The listing builds one solid part. Answer for the finished solid, in the listing's coordinates (mm). Face numbers are marked on the shaded views. A direction names the side the tool comes from. Coordinates: 2 decimals unless noted, no trailing zeros. Loops run counter-clockwise (first coordinate to the right, second up) from the corner with the lowest first, then second, coordinate; pieces in that order, holes last. Notation, with made-up numbers: (52, 12) - (94, 12) arc R23 ccw to (94, 34) - close; hole circle Ø5 at (28, -35). An arc over 180 degrees is marked (long way). Put each result on its own line as item: value.
```python
from build123d import *

# Parameters (mm, degrees)
BOSS_EXTRUDE1_DEPTH = 15.875


with BuildPart() as part:
    # Sketch1 → Boss-Extrude1 (new body)
    with BuildSketch(Plane.XY.offset(15.875)):
        with BuildLine():
            ThreePointArc((-3.888063673, 9.38661605), (-4.408258789, 9.153843698), (-4.914583893, 8.892269967))
            ThreePointArc((-4.914583893, 8.892269967), (-4.69950786, 7.393612219), (-4.22574714, 5.955633246))
            ThreePointArc((-4.22574714, 5.955633246), (-4.553034278, 5.709324401), (-4.865995885, 5.445051909))
            ThreePointArc((-4.865995885, 5.445051909), (-6.162500046, 6.226914882), (-7.575724395, 6.770081232))
            ThreePointArc((-7.575724395, 6.770081232), (-7.943407862, 6.334656387), (-8.286098429, 5.879300369))
            ThreePointArc((-8.286098429, 5.879300369), (-7.442078391, 4.622374388), (-6.391319038, 3.532357173))
            ThreePointArc((-6.391319038, 3.532357173), (-6.579325158, 3.168436005), (-6.746630286, 2.794545765))
            ThreePointArc((-6.746630286, 2.794545765), (-8.253977802, 2.93644789), (-9.762919991, 2.812648796))
            ThreePointArc((-9.762919991, 2.812648796), (-9.905267588, 2.260812689), (-10.016449548, 1.701863229))
            ThreePointArc((-10.016449548, 1.701863229), (-8.710654026, 0.93561862), (-7.291011817, 0.409454441))
            ThreePointArc((-7.291011817, 0.409454441), (-7.3025, 0), (-7.291011817, -0.409454441))
            ThreePointArc((-7.291011817, -0.409454441), (-8.710654026, -0.93561862), (-10.016449548, -1.701863229))
            ThreePointArc((-10.016449548, -1.701863229), (-9.905267588, -2.260812689), (-9.762919991, -2.812648796))
            ThreePointArc((-9.762919991, -2.812648796), (-8.253977802, -2.93644789), (-6.746630286, -2.794545765))
            ThreePointArc((-6.746630286, -2.794545765), (-6.579325158, -3.168436005), (-6.391319038, -3.532357173))
            ThreePointArc((-6.391319038, -3.532357173), (-7.442078391, -4.622374388), (-8.286098429, -5.879300369))
            ThreePointArc((-8.286098429, -5.879300369), (-7.943407862, -6.334656387), (-7.575724395, -6.770081232))
            ThreePointArc((-7.575724395, -6.770081232), (-6.162500046, -6.226914882), (-4.865995885, -5.445051909))
            ThreePointArc((-4.865995885, -5.445051909), (-4.553034278, -5.709324401), (-4.22574714, -5.955633246))
            ThreePointArc((-4.22574714, -5.955633246), (-4.69950786, -7.393612219), (-4.914583893, -8.892269967))
            ThreePointArc((-4.914583893, -8.892269967), (-4.408258789, -9.153843698), (-3.888063673, -9.38661605))
            ThreePointArc((-3.888063673, -9.38661605), (-2.850463577, -8.284065014), (-2.021591322, -7.017098744))
            ThreePointArc((-2.021591322, -7.017098744), (-1.62495912, -7.119411079), (-1.223214196, -7.199323113))
            ThreePointArc((-1.223214196, -7.199323113), (-1.026142161, -8.700454472), (-0.569675744, -10.144016441))
            ThreePointArc((-0.569675744, -10.144016441), (0, -10.16), (0.569675744, -10.144016441))
            ThreePointArc((0.569675744, -10.144016441), (1.026142161, -8.700454472), (1.223214196, -7.199323113))
            ThreePointArc((1.223214196, -7.199323113), (1.62495912, -7.119411079), (2.021591322, -7.017098744))
            ThreePointArc((2.021591322, -7.017098744), (2.850463577, -8.284065014), (3.888063673, -9.38661605))
            ThreePointArc((3.888063673, -9.38661605), (4.408258789, -9.153843698), (4.914583893, -8.892269967))
            ThreePointArc((4.914583893, -8.892269967), (4.69950786, -7.393612219), (4.22574714, -5.955633246))
            ThreePointArc((4.22574714, -5.955633246), (4.553034278, -5.709324401), (4.865995885, -5.445051909))
            ThreePointArc((4.865995885, -5.445051909), (6.162500046, -6.226914882), (7.575724395, -6.770081232))
            ThreePointArc((7.575724395, -6.770081232), (7.943407862, -6.334656387), (8.286098429, -5.879300369))
            ThreePointArc((8.286098429, -5.879300369), (7.442078391, -4.622374388), (6.391319038, -3.532357173))
            ThreePointArc((6.391319038, -3.532357173), (6.579325158, -3.168436005), (6.746630286, -2.794545765))
            ThreePointArc((6.746630286, -2.794545765), (8.253977802, -2.93644789), (9.762919991, -2.812648796))
            ThreePointArc((9.762919991, -2.812648796), (9.905267588, -2.260812689), (10.016449548, -1.701863229))
            ThreePointArc((10.016449548, -1.701863229), (8.710654026, -0.93561862), (7.291011817, -0.409454441))
            ThreePointArc((7.291011817, -0.409454441), (7.3025, 0), (7.291011817, 0.409454441))
            ThreePointArc((7.291011817, 0.409454441), (8.710654026, 0.93561862), (10.016449548, 1.701863229))
            ThreePointArc((10.016449548, 1.701863229), (9.905267588, 2.260812689), (9.762919991, 2.812648796))
            ThreePointArc((9.762919991, 2.812648796), (8.253977802, 2.93644789), (6.746630286, 2.794545765))
            ThreePointArc((6.746630286, 2.794545765), (6.579325158, 3.168436005), (6.391319038, 3.532357173))
            ThreePointArc((6.391319038, 3.532357173), (7.442078391, 4.622374388), (8.286098429, 5.879300369))
            ThreePointArc((8.286098429, 5.879300369), (7.943407862, 6.334656387), (7.575724395, 6.770081232))
            ThreePointArc((7.575724395, 6.770081232), (6.162500046, 6.226914882), (4.865995885, 5.445051909))
            ThreePointArc((4.865995885, 5.445051909), (4.553034278, 5.709324401), (4.22574714, 5.955633246))
            ThreePointArc((4.22574714, 5.955633246), (4.69950786, 7.393612219), (4.914583893, 8.892269967))
            ThreePointArc((4.914583893, 8.892269967), (4.408258789, 9.153843698), (3.888063673, 9.38661605))
            ThreePointArc((3.888063673, 9.38661605), (2.850463577, 8.284065014), (2.021591322, 7.017098744))
            ThreePointArc((2.021591322, 7.017098744), (1.62495912, 7.119411079), (1.223214196, 7.199323113))
            ThreePointArc((1.223214196, 7.199323113), (1.026142161, 8.700454472), (0.569675744, 10.144016441))
            ThreePointArc((0.569675744, 10.144016441), (0, 10.16), (-0.569675744, 10.144016441))
            ThreePointArc((-0.569675744, 10.144016441), (-1.026142161, 8.700454472), (-1.223214196, 7.199323113))
            ThreePointArc((-1.223214196, 7.199323113), (-1.62495912, 7.119411079), (-2.021591322, 7.017098744))
            ThreePointArc((-2.021591322, 7.017098744), (-2.850463577, 8.284065014), (-3.888063673, 9.38661605))
        make_face()
        with BuildLine():
            Line((1, 5), (1, 3.872983346))
            ThreePointArc((1, 3.872983346), (0, -4), (-1, 3.872983346))
            Line((-1, 3.872983346), (-1, 5))
            Line((-1, 5), (1, 5))
        make_face(mode=Mode.SUBTRACT)
    extrude(amount=-BOSS_EXTRUDE1_DEPTH)


solid = part.part
```
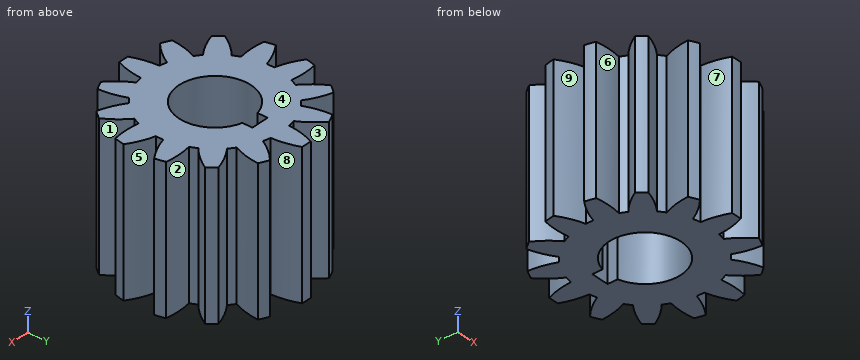
1) The part is cut by section D-D (y = -4.75). Give the vertices of the cut face in (x, z) (3 decimals).
Found:
outline: (-7.543, 0) - (7.543, 0) - (7.543, 15.875) - (-7.543, 15.875) - close
2) The part is cut by section C-C (x = -4.5). Give the vertices of the cut face in (y, z) (3 decimals).
Found:
outline: (-9.109, 0) - (-6.682, 0) - (-6.682, 15.875) - (-9.109, 15.875) - close; (-5.751, 0) - (5.751, 0) - (5.751, 15.875) - (-5.751, 15.875) - close; (6.682, 0) - (9.109, 0) - (9.109, 15.875) - (6.682, 15.875) - close
3) For a pull along Y with two mould halves and no side action, classify the marked faces 1, 2, 3 and 4 as pulls with the +Y half, pulls with the -Y half, needs draft (parallel to the pull), parting line crosses it, or undercut.
Found:
face 1: undercut
face 2: undercut
face 3: pulls with the +Y half
face 4: needs draft
4) The part is cut by section A-A (x = 0). Give the vertices of the cut face in (y, z) (3 decimals), and give its area (3 significant figures).
Found:
outline: (-10.16, 0) - (-4, 0) - (-4, 15.875) - (-10.16, 15.875) - close; (5, 0) - (10.16, 0) - (10.16, 15.875) - (5, 15.875) - close
area: 180 mm^2
5) The part is cut by section B-B (y = 0). Give the vertices of the cut face in (x, z) (1 decimal).
Found:
outline: (-7.3, 0) - (-4, 0) - (-4, 15.9) - (-7.3, 15.9) - close; (4, 0) - (7.3, 0) - (7.3, 15.9) - (4, 15.9) - close
6) Straight lines are drawn through the part: L1, parallel to X at y = -7.25, z = 4.5; L2, parallel to Y at x = 8.5, z = 11.75; L3, parallel to Y at x = 3.5, z = 7. For each, find the intervals that lie inside material, in ascending order. Write a range as [from, to].
Found:
L1: x = [-4.66, -2.15], [-1.22, 1.22], [2.15, 4.66]
L2: y = [-2.93, -0.84], [0.84, 2.93]
L3: y = [-9.02, -1.94], [1.94, 9.02]
7) For the marked faces 5, 6, 7, 8 and 9, determine the directions among +Z, -Z, +X, -X, +Y, -Y from which every point of the face is accessible in a straight line to the end or side of a thin tool.
Found:
face 5: +Z, -Z, +X
face 6: +Z, -Z
face 7: +Z, -Z, -Y
face 8: +Z, -Z, +Y
face 9: +Z, -Z, -X
8) Each of these flat-tipped pins is pushed along its axis until it touches: pin 1 (0.6 mm diameter, centred on y = 4.5, z = 11, fed in from +X); pin 2 (1.5 mm diameter, centred on x = 4.5, z = 10, fed in from +Y); pin 3 (1.5 mm diameter, centred on y = -7, z = 13, fed in from -X); pin 4 (7 mm diameter, centred on x = 0, y = 0, fed in from +Z). Where does it stop, or does it pass through?
Found:
pin 1: stops at x = 7.58
pin 2: stops at y = 9.39
pin 3: stops at x = -8.01
pin 4: passes through
